The model under review builds one solid part; all positions refer to its coordinate system, in mm. A direction names the side the tool comes from. Give positions to 0.01 mm unless a question says otherwise; leave off trailing zeros. Loops run counter-clockwise (first coordinate to the right, second up) from the corner with the lowest first, then second, coordinate; pieces in that order, holes last. Notation, with made-up numbers: M -9.5,56.5 L -3.5,56.5 A16 ccw -3.5,61.5 Z; hole C 11,5 d5. An arc over 180 degrees is marked long. One line per item, written item: value. Start each with the question number.
Q1. We need section C-C on x = 43. Write out the cut boundary in (y, z).
Q2. We need section A-A on z = 0. Write out the cut boundary in (x, y), plus the area to 3 significant figures.
Q3. To check wall thickness, follow line 1 along Z through (x, y) = (0, -97.75); line 2 along Z through (x, y) = (0, -42); line 3 along Z through (x, y) = (0, -168). State the ranges of each line that lie inside material, in increasing order. Write a range as from..to.
Q4. Mouldability with a two-part tool opening along Z and no side actions: class faces 3 (the face through (49, -161, 15)), 4 (the face through (-90.97, -100.18, -69.75)), 5 (the face through (49, -203.2, -24)) as released by +Z, released by -Z, zero draft, split by the parting line, or undercut.
Q5. For faces 1 (the face through (-15, -117.856, 34)), 2 (the face through (-29.227, -59.753, -22.41)), list the 3-axis set-ups (+Z, -Z, +X, -X, +Y, -Y) from which the entire face can be reached by the end or side of a thin tool; tool diameter is ignored.
Q6. For pin 1 (1 mm diameter, centred on x = 55.5, y = -153.5, fed in from -Z); pin 2 (1 mm diameter, centred on x = -44.5, y = -72.5, fed in from -Z); pin 3 (12 mm diameter, centred on x = -31.5, z = -91, fed in from +Y); pin 4 (2.5 mm diameter, centred on x = 0, z = -45.5, fed in from -Y), all flat-tipped, find the tip position at first contact; note any pin that passes through.
Q7. We need section B-B on y = -105.5. Write out the cut boundary in (x, z).
Q8. We need section D-D on y = -164.5. Write out the cut boundary in (x, z).
```python
from build123d import *

# Parameters (mm, degrees)
F0_R     = 114.633929
F1_DEPTH = 203.2
F2_R     = 36.83
F3_DEPTH = 355.6
F4_R     = 51.2445
F5_DEPTH = 85.344
F6_R     = 2.6289
F7_DEPTH = 28.575


with BuildPart() as f1:
    # F0 (on Front) → F1 (new body)
    with BuildSketch(Plane.XZ):
        Circle(F0_R)
    extrude(amount=F1_DEPTH)

    # F2 (on face) → F3 (cut)
    with BuildSketch(Plane.XZ.offset(203.2)):
        Circle(F2_R)
    extrude(amount=-F3_DEPTH, mode=Mode.SUBTRACT)

    # F4 (on face) → F5 (cut)
    with BuildSketch(Plane.XZ.offset(203.2)):
        Circle(F4_R)
    extrude(amount=-F5_DEPTH, mode=Mode.SUBTRACT)

    # F6 (on face) → F7 (cut)
    with BuildSketch(Plane.XZ.offset(117.856)):
        with Locations((0, -44.45)):
            Circle(F6_R)
    extrude(amount=-F7_DEPTH, mode=Mode.SUBTRACT)


solid = f1.part
```
Solved:
1. outline: M -203.2,-106.26 L 0,-106.26 L 0,106.26 L -203.2,106.26 L -203.2,27.87 L -117.86,27.87 L -117.86,-27.87 L -203.2,-27.87 Z
2. outline: M -114.63,-203.2 L -51.24,-203.2 L -51.24,-117.86 L -36.83,-117.86 L -36.83,0 L -114.63,0 Z; M 36.83,-117.86 L 51.24,-117.86 L 51.24,-203.2 L 114.63,-203.2 L 114.63,0 L 36.83,0 Z
2. area: 29,200 mm2
3. line 1: -114.63..-47.08, -41.82..-36.83, 36.83..114.63
3. line 2: -114.63..-36.83, 36.83..114.63
3. line 3: -114.63..-51.24, 51.24..114.63
4. face 3: undercut
4. face 4: split by the parting line
4. face 5: zero draft
5. face 1: -Y
5. face 2: +Y, -Y
6. pin 1: z = -100.58
6. pin 2: z = -105.85
6. pin 3: y = 0
6. pin 4: y = -89.28
7. outline: C 0,0 d229.27; hole C 0,0 d73.66; hole C 0,-44.45 d5.26
8. outline: C 0,0 d229.27; hole C 0,0 d102.49
